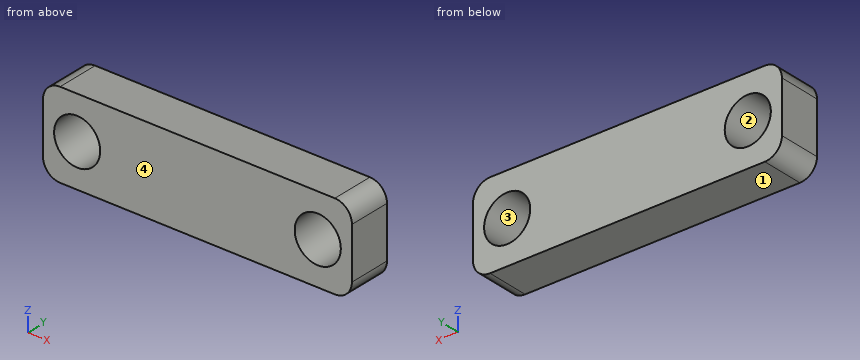
from build123d import *

# Parameters (mm, degrees)
SKETCH1_W              = 18.09
SKETCH1_H              = 5
BOSS_EXTRUDE1_DEPTH    = 2.5
M2_5_CLEARANCE_HOLE1_D = 2.7
FILLET1_R              = 1


with BuildPart() as part:
    # Sketch1 → Boss-Extrude1 (new body)
    with BuildSketch(Plane(origin=(0, 0, 0), x_dir=(1, 0, 0), z_dir=(0, 1, 0))):
        Rectangle(SKETCH1_W, SKETCH1_H)
    extrude(amount=BOSS_EXTRUDE1_DEPTH)

    # M2.5 Clearance Hole1 (through all)
    with Locations(Plane(origin=(0, 0, 0), x_dir=(-1, 0, 0), z_dir=(0, -1, 0))):
        with Locations((-7.045, 0), (7.045, 0)):
            Hole(M2_5_CLEARANCE_HOLE1_D / 2)

    # Fillet1
    fillet1_edges = [part.edges().sort_by_distance(p)[0] for p in [
        (9.045, 1.25, 2.5),
        (-9.045, 1.25, 2.5),
        (-9.045, 1.25, -2.5),
        (9.045, 1.25, -2.5),
    ]]
    fillet(fillet1_edges, radius=FILLET1_R)


solid = part.part
Build history of the part. All positions in model axes, mm. Face numbers are marked on the shaded views. Give positions to 0.01 mm unless a question says otherwise; leave off trailing zeros. Loops run counter-clockwise (first coordinate to the right, second up) from the corner with the lowest first, then second, coordinate; pieces in that order, holes last. Notation, with made-up numbers: (75.5, -11.75) - (126.5, -11.75) arc R15 cw to (126.5, 17.25) - close; hole circle Ø11 at (-6.5, 52.25). An arc over 180 degrees is marked (long way). Write item = value, one per line. Start each with the question number.
1) Probe probe 1 along X at (y, z) = (2.15, -0.05) (3 decimals); probe 2 along X at (y, z) = (2.4, -1.15) (3 decimals); probe 3 along Z at (x, y) = (-7, 0.9). List the from-to ranges inside material, lowest first. Write a range as from..to.
2) Band-saw the part on B-B on z = 0. Give the cut face in (x, y) (3 decimals), plus the area to 3 significant figures.
3) Band-saw the part on C-C on x = 7. Give the cut face in (y, z), plus the area to 3 significant figures.
4) Drop a flat-ended pin along its axis: pin 1 Ø2 at (x, z) = (-7.045, 0) entering from -Y. Give the stop position or say it passes through.
5) Band-saw the part on A-A on y = 1.4. Give the cut face in (x, z) (3 decimals).
6) Band-saw the part on D-D on z = -1.1. Give the cut face in (x, y) (3 decimals), plus the area to 3 significant figures.
7) Pull direction Z, two halves, no side cores. Call the marked faces 1, 2, 3 and 4: +Z half, -Z half, draft (parallel to the pull), parting line (faces both ways), or undercut.
Final values:
q1.probe_1 = -9.045..-8.394, -5.696..5.696, 8.394..9.045
q1.probe_2 = -9.045..-7.752, -6.338..6.338, 7.752..9.045
q1.probe_3 = -2.5..-1.35, 1.35..2.5
q2.outline = (-9.045, 0) - (-8.395, 0) - (-8.395, 2.5) - (-9.045, 2.5) - close; (-5.695, 0) - (5.695, 0) - (5.695, 2.5) - (-5.695, 2.5) - close; (8.395, 0) - (9.045, 0) - (9.045, 2.5) - (8.395, 2.5) - close
q2.area = 31.7 mm²
q3.outline = (0, -2.5) - (2.5, -2.5) - (2.5, -1.35) - (0, -1.35) - close; (0, 1.35) - (2.5, 1.35) - (2.5, 2.5) - (0, 2.5) - close
q3.area = 5.75 mm²
q4.pin_1 = through
q5.outline = (-9.045, -1.5) arc R1 ccw to (-8.045, -2.5) - (8.045, -2.5) arc R1 ccw to (9.045, -1.5) - (9.045, 1.5) arc R1 ccw to (8.045, 2.5) - (-8.045, 2.5) arc R1 ccw to (-9.045, 1.5) - close; hole circle Ø2.7 at (-7.045, 0); hole circle Ø2.7 at (7.045, 0)
q6.outline = (-9.045, 0) - (-7.828, 0) - (-7.828, 2.5) - (-9.045, 2.5) - close; (-6.262, 0) - (6.262, 0) - (6.262, 2.5) - (-6.262, 2.5) - close; (7.828, 0) - (9.045, 0) - (9.045, 2.5) - (7.828, 2.5) - close
q6.area = 37.4 mm²
q7.face_1 = -Z half
q7.face_2 = undercut
q7.face_3 = undercut
q7.face_4 = draft
